Source: CAD feature listing. Evaluate the final solid. Frame: model axes, mm. A direction names the side the tool comes from. Round coordinates to 2 decimals unless told otherwise and drop trailing zeros. Order: outer loops, then holes, each group sorted by start corner. A loop starts at its lowest first (then second) coordinate and runs counter-clockwise, first axis right, second up. Notation, with made-up numbers: M 81.5,58 L 102.5,58 A21 cw 102.5,72 Z; hole C -8,48.25 d2. An arc over 180 degrees is marked long. Answer as CSV lines item,"result". Start each with the question number.
Item 1: Section query B-B on x = 76.2. Return the cut outline in (y, z) (3 decimals).
Item 2: Section query A-A on y = 38.1. Return the cut outline in (x, z) (3 decimals), plus the area to 3 significant figures.
Item 3: Line query: line 1 (Y direction, x = 76.2, z = 8.75); line 2 (Y direction, x = 76.2, z = 3); line 3 (Z direction, x = 95, y = 69). Output: solid intervals per line, ascending. Write a range as [from, to].
Item 4: Section query C-C on y = 21.5. Return the cut outline in (x, z) (3 decimals), plus the area to 3 significant figures.
Item 5: Section query D-D on x = 34.5. Return the cut outline in (y, z) (3 decimals), plus the area to 3 significant figures.
Item 6: Set-up query: faces 1 (the face through (69, 63, 6.35)), 2 (the face through (55, 101.6, 3)). Return all of +Z, -Z, +X, -X, +Y, -Y with unobstructed straight access to the full face (end or side cutting, diameter ignored); none if empty.
Item 7: First-contact query: P1, Ø4, axis at x = 115, y = 82, coming from the -Z side; P2, Ø1.5, axis at x = 103.5, y = 34, coming from the +Z side. Flat tips, straight axial feed; report the tip coordinate or a pass-through.
Item 8: Pull-direction query (X, two-part tool) for faces 3 (the face through (70, 50, 9.525)), 4 (the face through (139.7, 25, 3)), 5 (the face through (12.712, 64.058, 7.915)); classes: +X half, -X half, draft (parallel to the pull), parting line (faces both ways), or undercut.
from build123d import *

# Parameters (mm, degrees)
BOSS_EXTRUDE2_DEPTH = 6.35
SKETCH2_R           = 12.7
SKETCH2_R_2         = 25.4
BOSS_EXTRUDE4_DEPTH = 3.175
SKETCH5_R           = 12.7
CUT_EXTRUDE1_DEPTH  = 127


with BuildPart() as part:
    # Sketch1 → Boss-Extrude2 (new body)
    with BuildSketch(Plane.XY):
        Polygon((0, 0), (139.7, 0), (139.7, 50.8), (107.95, 101.6), (0, 101.6), align=None)
    extrude(amount=BOSS_EXTRUDE2_DEPTH)

    # Sketch2 → Boss-Extrude4 (add)
    with BuildSketch(Plane.XY.offset(6.35)):
        with Locations((25.4, 63.5)):
            Circle(SKETCH2_R)
        with Locations((76.2, 38.1)):
            Circle(SKETCH2_R_2)
        with Locations((76.2, 38.1)):
            Circle(SKETCH2_R, mode=Mode.SUBTRACT)
    extrude(amount=BOSS_EXTRUDE4_DEPTH)

    # Sketch5 → Cut-Extrude1 (cut)
    with BuildSketch(Plane.XY.offset(6.35)):
        with Locations((76.2, 38.1)):
            Circle(SKETCH5_R)
    extrude(amount=-CUT_EXTRUDE1_DEPTH, mode=Mode.SUBTRACT)


solid = part.part
Results:
1,outline,"M 0,0 L 25.4,0 L 25.4,9.525 L 12.7,9.525 L 12.7,6.35 L 0,6.35 Z; M 50.8,0 L 101.6,0 L 101.6,6.35 L 63.5,6.35 L 63.5,9.525 L 50.8,9.525 Z"
2,outline,"M 0,0 L 63.5,0 L 63.5,9.525 L 50.8,9.525 L 50.8,6.35 L 0,6.35 Z; M 88.9,0 L 139.7,0 L 139.7,6.35 L 101.6,6.35 L 101.6,9.525 L 88.9,9.525 Z"
2,area,"806 mm^2"
3,line 1,"[12.7, 25.4], [50.8, 63.5]"
3,line 2,"[0, 25.4], [50.8, 101.6]"
3,line 3,"[0, 6.35]"
4,outline,"M 0,0 L 139.7,0 L 139.7,6.35 L 95.425,6.35 L 95.425,9.525 L 56.975,9.525 L 56.975,6.35 L 0,6.35 Z"
4,area,"1,010 mm^2"
5,outline,"M 0,0 L 101.6,0 L 101.6,6.35 L 72.359,6.35 L 72.359,9.525 L 54.641,9.525 L 54.641,6.35 L 0,6.35 Z"
5,area,"701 mm^2"
6,face 1,"+Z"
6,face 2,"+Z, -Z, +X, -X, +Y"
7,P1,"z = 0"
7,P2,"z = 6.35"
8,face 3,"draft"
8,face 4,"+X half"
8,face 5,"undercut"
